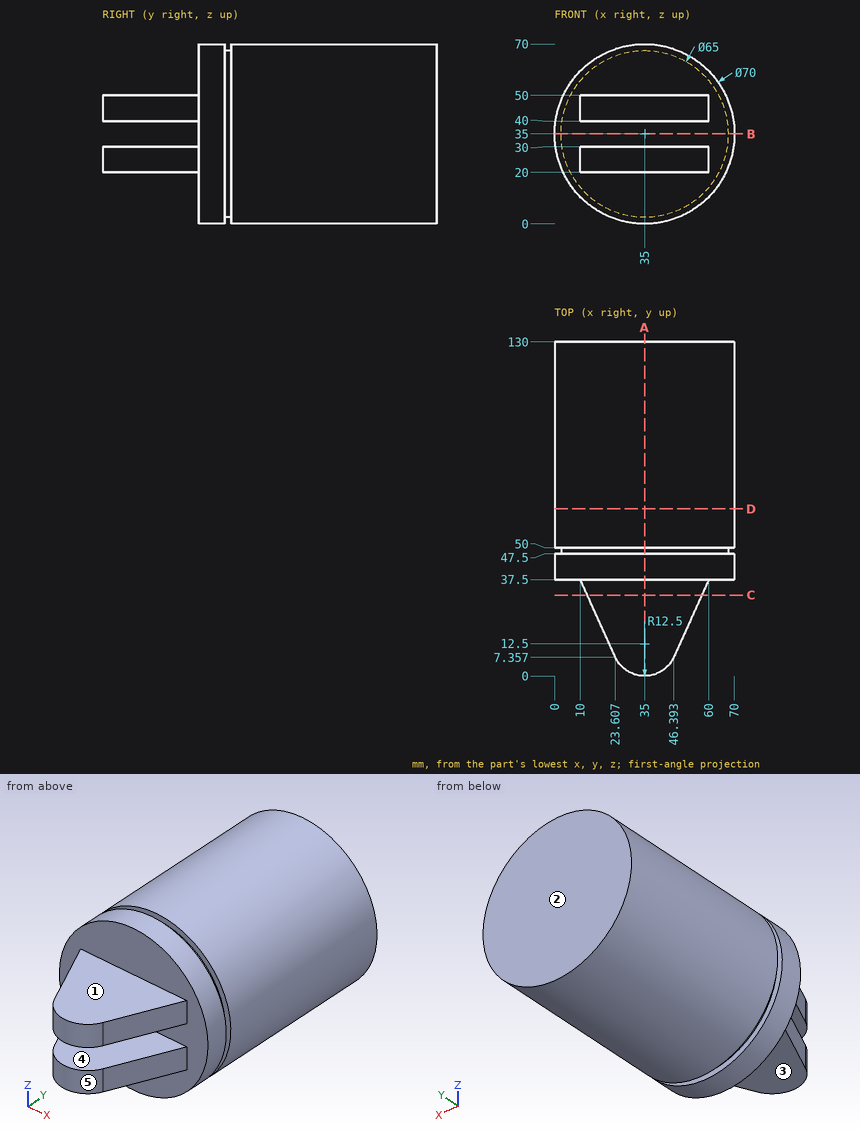
For this review, use the dimensioned drawing (mm, ordinates from the lowest corner) and the shaded views. A direction names the side the tool comes from. Coordinates: 2 decimals unless noted, no trailing zeros. Write each loop counter-clockwise with the first axis right and the second up, starting at its lowest first coordinate (ties: lowest second). Pieces come first, ordered by that corner, then holes. Notation, with made-up numbers: (41.5, -11) -> (63.5, -11) arc R12 ccw to (63.5, -2) -> close; hole circle Ø1 at (62.5, -22). An arc over 180 degrees is marked (long way). Write each question's results on one line, items separated by ' | '. Start each with the question number.
(1) The part is to be moulded in two halves that separate along Z. For the marked faces 3, 4 and 5, say which applies: pulls with the +Z half, pulls with the -Z half, needs draft (parallel to the pull), parting line crosses it, or undercut.
(2) Take a section at C-C on y = 31.5. Write out the cut boundary in (x, z), and give its area (3 significant figures).
(3) Take a section at A-A on x = 35. Write out the cut boundary in (y, z).
(4) Take a section at B-B on z = 35. Write out the cut boundary in (x, y), and give its area (3 significant figures).
(5) Take a section at D-D on y = 65. Write out the cut boundary in (x, z).
(6) For line 1 along Y through (x, z) = (66.5, 24.5); line 2 along Z through (x, y) = (35, 9); line 3 along Y through (x, z) = (63.5, 38), list the stretches that pass through material, from the lowest coordinate up. Write a range as from..to.
(7) Clearance check with flat-ended pins moving along their axes: P1, Ø11, axis at x = 26, y = 17.5, coming from the +Z side; P2, Ø5, axis at y = 13.5, z = 27.5, coming from the -X side; P3, Ø6, axis at y = 67.5, z = 63, coming from the +X side (3 decimals). State where each tip first meets the part, or that it passes through.
(8) Tool access review of the marked faces 1 and 2: name each direction out of +Z, -Z, +X, -X, +Y, -Y from which nothing blocks a thin tool from reaching the whole face with its end or side.
Results found:
1) face 3: pulls with the -Z half | face 4: undercut | face 5: needs draft
2) outline: (12.71, 20) -> (57.29, 20) -> (57.29, 30) -> (12.71, 30) -> close; (12.71, 40) -> (57.29, 40) -> (57.29, 50) -> (12.71, 50) -> close | area: 892 mm2
3) outline: (0, 20) -> (37.5, 20) -> (37.5, 0) -> (47.5, 0) -> (47.5, 2.5) -> (50, 2.5) -> (50, 0) -> (130, 0) -> (130, 70) -> (50, 70) -> (50, 67.5) -> (47.5, 67.5) -> (47.5, 70) -> (37.5, 70) -> (37.5, 50) -> (0, 50) -> (0, 40) -> (37.5, 40) -> (37.5, 30) -> (0, 30) -> close
4) outline: (0, 37.5) -> (70, 37.5) -> (70, 47.5) -> (67.5, 47.5) -> (67.5, 50) -> (70, 50) -> (70, 130) -> (0, 130) -> (0, 50) -> (2.5, 50) -> (2.5, 47.5) -> (0, 47.5) -> close | area: 6,460 mm2
5) outline: circle Ø70 at (35, 35)
6) line 1: y = 37.5..47.5, 50..130 | line 2: z = 20..30, 40..50 | line 3: y = 37.5..130
7) P1: stops at z = 50 | P2: stops at x = 19.71 | P3: stops at x = 59.495
8) face 1: +Z, +X, -X, -Y | face 2: +Z, -Z, +X, -X, +Y
